Could you check a few things on this model? Use its own coordinates, in mm. A direction names the side the tool comes from. Give positions to 0.01 mm unless a question says otherwise; leave off trailing zeros. Write each loop counter-clockwise with the first axis right and the second up, starting at its lowest first coordinate (ties: lowest second). Pieces come first, ordered by that corner, then holes. Notation, with made-up numbers: (77, -33) -> (88, -33) arc R12 ccw to (88, -14) -> close; hole circle Ø2 at (-37.75, 52). An arc over 180 degrees is marked (long way). One line per question, with ' | ' between items.
from build123d import *

# Parameters (mm, degrees)
F0_W      = 500
F0_H      = 300
F1_DEPTH  = 400
F2_W      = 194.6479137987
F2_H      = 116.2542514503
F2_W_2    = 185.7395432889
F2_H_2    = 104.6733558178
F3_DEPTH  = 200
F4_W      = 200.438356027
F4_H      = 251.2160688639
F4_W_2    = 207.3423415422
F4_H_2    = 244.5347867906
F5_DEPTH  = 200
F6_W      = 311.2314343452
F6_H      = 161.7837399244
F7_DEPTH  = 300
F8_W      = 785.5169922113
F8_H      = 196.2788403034
F9_DEPTH  = 200
F10_DEPTH = 200
F11_W     = 207.3423415422
F11_H     = 178.8012206554
F12_DEPTH = 300
F13_W     = 330.7198137045
F13_H     = 196.2788403034
F14_DEPTH = 700
F15_W     = 178.8012206554
F15_H     = 229.1771650314
F16_DEPTH = 400
F17_W     = 166.0685539246
F17_H     = 392.9448246956
F18_DEPTH = 200
F19_DEPTH = 600
F20_W     = 166.0685539246
F20_H     = 228.0832886696
F21_DEPTH = 230
F22_W     = 230
F22_H     = 228.0832886696
F23_DEPTH = 600
F24_W     = 191.9558256865
F24_H     = 228.0832886696
F25_DEPTH = 600
F26_W     = 330.7198137045
F26_H     = 224.4375318289
F27_DEPTH = 500
F28_W     = 330.7198137045
F28_H     = 150.941491127
F29_DEPTH = 400
F30_W     = 330.7198137045
F30_H     = 173.616194725
F31_DEPTH = 300
F32_W     = 230.9049870819
F32_H     = 232.3303222656
F33_DEPTH = 400
F34_W     = 200
F34_H     = 232.3303222656
F35_DEPTH = 400
F36_W     = 134.3211080879
F36_H     = 232.3303222656
F37_DEPTH = 450
F38_W     = 220.0524806976
F38_H     = 194.8631778359
F39_DEPTH = 1000
F40_W     = 194.8631778359
F40_H     = 226.6708314419
F41_DEPTH = 500
F42_W     = 213.9312028885
F42_H     = 194.8631778359
F43_DEPTH = 300
F44_W     = 213.9312028885
F44_H     = 224.6371984482
F45_DEPTH = 150
F46_W     = 172.431588918
F46_H     = 224.6371984482
F47_DEPTH = 400
F48_R     = 65.9786612065
F49_DEPTH = 100
F50_R     = 50
F51_DEPTH = 100
F52_R     = 50
F53_DEPTH = 200
F54_R     = 50
F55_DEPTH = 200
F56_R     = 50
F57_DEPTH = 200
F58_W     = 1393.2492136955
F58_H     = 511.3118588924
F58_R     = 50
F59_DEPTH = 200


with BuildPart() as f1:
    # F0 (on Front) → F1 (new body)
    with BuildSketch(Plane.XZ):
        with Locations((0, -50)):
            Rectangle(F0_W, F0_H)
    extrude(amount=F1_DEPTH)

    # F2 (on face) → F3 (join)
    with BuildSketch(Plane.XY.offset(100)):
        with Locations((110.0183846429, -98.0239007622)):
            Rectangle(F2_W, F2_H)
        with Locations((-118.4813398868, -227.6407033205)):
            Rectangle(F2_W_2, F2_H_2)
    extrude(amount=F3_DEPTH)

    # F4 (on face) → F5 (join)
    with BuildSketch(Plane.XY.offset(300)):
        with Locations((-111.1319335178, -154.3693467975)):
            Rectangle(F4_W, F4_H)
        with Locations((103.6711707711, -161.2733323127)):
            Rectangle(F4_W_2, F4_H_2)
    extrude(amount=F5_DEPTH)

    # F6 (on face) → F7 (join)
    with BuildSketch(Plane.XZ.offset(400)):
        with Locations((3.1632035971, -80.8918699622)):
            Rectangle(F6_W, F6_H)
    extrude(amount=F7_DEPTH)

    # F8 (on face) → F9 (join)
    with BuildSketch(Plane(origin=(0, -28.7613123655, 0), x_dir=(-1, 0, 0), z_dir=(0, 1, 0))):
        with Locations((-181.4073845744, 401.8605798483)):
            Rectangle(F8_W, F8_H)
    extrude(amount=F9_DEPTH)

    # F10 (add): a face of the model
    f10_faces = [f1.faces().sort_by_distance(p)[0] for p in [
        (103.6711707711, -283.540725708, 400),
    ]]
    extrude(f10_faces, amount=F10_DEPTH)

    # F11 (on face) → F12 (join)
    with BuildSketch(Plane.XY.offset(500)):
        with Locations((103.6711707711, -394.1401153803)):
            Rectangle(F11_W, F11_H)
    extrude(amount=F12_DEPTH)

    # F13 (on face) → F14 (join)
    with BuildSketch(Plane.XZ.offset(28.7613123655)):
        with Locations((408.8059738278, 401.8605798483)):
            Rectangle(F13_W, F13_H)
    extrude(amount=F14_DEPTH)

    # F15 (on face) → F16 (join)
    with BuildSketch(Plane.YZ.offset(207.3423415422)):
        with Locations((-394.1401153803, 685.4114174843)):
            Rectangle(F15_W, F15_H)
    extrude(amount=F16_DEPTH)

    # F17 (on face) → F18 (join)
    with BuildSketch(Plane(origin=(-250, 0, 0), x_dir=(0, -1, 0), z_dir=(-1, 0, 0))):
        with Locations((368.2630956173, -3.5275876522)):
            Rectangle(F17_W, F17_H)
    extrude(amount=F18_DEPTH)

    # F19 (add): a face of the model
    f19_faces = [f1.faces().sort_by_distance(p)[0] for p in [
        (-350, -368.2630956173, 192.9448246956),
    ]]
    extrude(f19_faces, amount=F19_DEPTH)

    # F20 (on face) → F21 (join)
    with BuildSketch(Plane.YZ.offset(-250)):
        with Locations((-368.2630956173, 678.9031803608)):
            Rectangle(F20_W, F20_H)
    extrude(amount=F21_DEPTH)

    # F22 (on face) → F23 (join)
    with BuildSketch(Plane(origin=(0, -285.228818655, 0), x_dir=(-1, 0, 0), z_dir=(0, 1, 0))):
        with Locations((135, 678.9031803608)):
            Rectangle(F22_W, F22_H)
    extrude(amount=F23_DEPTH)

    # F24 (on face) → F25 (join)
    with BuildSketch(Plane.YZ.offset(-20)):
        with Locations((218.7932685018, 678.9031803608)):
            Rectangle(F24_W, F24_H)
    extrude(amount=F25_DEPTH)

    # F26 (on face) → F27 (join)
    with BuildSketch(Plane.XY.offset(500)):
        with Locations((408.8059738278, -616.5425464511)):
            Rectangle(F26_W, F26_H)
    extrude(amount=F27_DEPTH)

    # F28 (on face) → F29 (join)
    with BuildSketch(Plane(origin=(0, -504.3237805367, 0), x_dir=(-1, 0, 0), z_dir=(0, 1, 0))):
        with Locations((-408.8059738278, 924.5292544365)):
            Rectangle(F28_W, F28_H)
    extrude(amount=F29_DEPTH)

    # F30 (on face) → F31 (join)
    with BuildSketch(Plane(origin=(0, 0, 849.058508873), x_dir=(1, 0, 0), z_dir=(0, 0, -1))):
        with Locations((408.8059738278, 191.1318778992)):
            Rectangle(F30_W, F30_H)
    extrude(amount=F31_DEPTH)

    # F32 (on face) → F33 (join)
    with BuildSketch(Plane(origin=(0, 0, 0), x_dir=(-1, 0, 0), z_dir=(0, 1, 0))):
        with Locations((-95.0625883415, -42.5678789616)):
            Rectangle(F32_W, F32_H)
    extrude(amount=F33_DEPTH)

    # F34 (on face) → F35 (join)
    with BuildSketch(Plane(origin=(-20.3899051994, 0, 0), x_dir=(0, -1, 0), z_dir=(-1, 0, 0))):
        with Locations((-300, -42.5678789616)):
            Rectangle(F34_W, F34_H)
    extrude(amount=F35_DEPTH)

    # F36 (on face) → F37 (join)
    with BuildSketch(Plane.XZ.offset(-200)):
        with Locations((-353.2293511555, -42.5678789616)):
            Rectangle(F36_W, F36_H)
    extrude(amount=F37_DEPTH)

    # F38 (on face) → F39 (join)
    with BuildSketch(Plane.XY.offset(73.5972821712)):
        with Locations((-396.0950374603, -152.568411082)):
            Rectangle(F38_W, F38_H)
    extrude(amount=F39_DEPTH)

    # F40 (on face) → F41 (join)
    with BuildSketch(Plane.YZ.offset(-286.0687971115)):
        with Locations((-152.568411082, 960.2618664503)):
            Rectangle(F40_W, F40_H)
    extrude(amount=F41_DEPTH)

    # F42 (on face) → F43 (join)
    with BuildSketch(Plane(origin=(0, 0, 846.9264507294), x_dir=(1, 0, 0), z_dir=(0, 0, -1))):
        with Locations((106.9656014442, 152.568411082)):
            Rectangle(F42_W, F42_H)
    extrude(amount=F43_DEPTH)

    # F44 (on face) → F45 (join)
    with BuildSketch(Plane(origin=(0, -55.1368221641, 0), x_dir=(-1, 0, 0), z_dir=(0, 1, 0))):
        with Locations((-106.9656014442, 659.2450499535)):
            Rectangle(F44_W, F44_H)
    extrude(amount=F45_DEPTH)

    # F46 (on face) → F47 (join)
    with BuildSketch(Plane.YZ.offset(213.9312028885)):
        with Locations((8.647383377, 659.2450499535)):
            Rectangle(F46_W, F46_H)
    extrude(amount=F47_DEPTH)

    # F48 (on face) → F49 (join)
    with BuildSketch(Plane.XZ.offset(700)):
        with Locations((0, -72.7314278483)):
            Circle(F48_R)
    extrude(amount=F49_DEPTH)

    # F50 (on face) → F51 (join)
    with BuildSketch(Plane.YZ.offset(607.3423415422)):
        with Locations((-393.540725708, 680)):
            Circle(F50_R)
    extrude(amount=F51_DEPTH)

    # F52 (on face) → F53 (join)
    with BuildSketch(Plane.YZ.offset(574.1658806801)):
        with Locations((-191.1318778992, 680)):
            Circle(F52_R)
    extrude(amount=F53_DEPTH)

    # F54 (on face) → F55 (join)
    with BuildSketch(Plane.YZ.offset(613.9312028885)):
        with Locations((8.647383377, 680)):
            Circle(F54_R)
    extrude(amount=F55_DEPTH)

    # F56 (on face) → F57 (join)
    with BuildSketch(Plane.YZ.offset(580)):
        with Locations((218.7932685018, 678.9031803608)):
            Circle(F56_R)
    extrude(amount=F57_DEPTH)

    # F58 (on face) → F59 (cut)
    with BuildSketch(Plane.YZ.offset(707.3423415422)):
        with Locations((-61.5827143192, 670.519605279)):
            Rectangle(F58_W, F58_H)
        with Locations((-393.540725708, 680)):
            Circle(F58_R, mode=Mode.SUBTRACT)
    extrude(amount=F59_DEPTH, mode=Mode.SUBTRACT)


solid = f1.part
Q1. Imagine slicing it at B-B on y = 143.5. Please give me the cut outline in (x, z), and give its area (3 significant figures).
Answer below:
outline: (-420.39, -158.73) -> (-286.07, -158.73) -> (-286.07, 73.6) -> (-420.39, 73.6) -> close; (-250, 564.86) -> (580, 564.86) -> (580, 792.94) -> (-250, 792.94) -> close; (-211.35, 303.72) -> (574.17, 303.72) -> (574.17, 500) -> (-211.35, 500) -> close; (-20.39, -158.73) -> (210.52, -158.73) -> (210.52, 73.6) -> (-20.39, 73.6) -> close | area: 428,000 mm^2
Q2. On a 3-axis mill with a long thin cutter (end or side, diameter ignored), from which of +Z, -Z, +X, -X, +Y, -Y can I reach the whole of each face in a straight line? I mean faces 1 (the flat face through (-3, -197, 100)), 2 (the flat face through (-250, -386, 262)), 3 (the flat face through (411, -421, 1000)), 4 (the cylindrical face through (659.983, 2.138, 729.575)), 5 (the flat face through (234, -42, 546.926)). Say none if no direction works.
Answer below:
face 1: none | face 2: -Y | face 3: +Z, +X, +Y, -Y | face 4: +X | face 5: +X, +Y
Q3. If we mould it in two halves opening along Y, with no side actions, what happens to faces 6 (the flat face through (102, -39.006, 399)), 7 (the flat face through (-113, -279.977, 297)), 8 (the flat face through (0, -314, 491))? For each: +Y half, -Y half, draft (parallel to the pull), parting line (faces both ways), or undercut.
Answer below:
face 6: undercut | face 7: -Y half | face 8: draft
Q4. Imagine slicing it at A-A on x = -108. Please give me the cut outline in (y, z).
Answer below:
outline: (-700, -161.78) -> (-400, -161.78) -> (-400, -200) -> (0, -200) -> (0, 100) -> (-175.3, 100) -> (-175.3, 300) -> (-28.76, 300) -> (-28.76, 303.72) -> (171.24, 303.72) -> (171.24, 500) -> (-279.98, 500) -> (-279.98, 100) -> (-400, 100) -> (-400, 0) -> (-700, 0) -> close; (-451.3, 564.86) -> (314.77, 564.86) -> (314.77, 792.94) -> (-451.3, 792.94) -> close; (-250, 846.93) -> (-55.14, 846.93) -> (-55.14, 1073.6) -> (-250, 1073.6) -> close; (200, -158.73) -> (400, -158.73) -> (400, 73.6) -> (200, 73.6) -> close
Q5. Will these pins go through, and if not, where does the flat tip stop? pin 1 (6 mm diameter, centred on x = 107.5, y = 250.5, fed in from +Z); pin 2 (2 mm diameter, centred on x = -115.5, z = 77, fed in from -Y); pin 3 (3 mm diameter, centred on x = -302, z = 349, fed in from +Y).
Answer below:
pin 1: stops at z = 792.94 | pin 2: stops at y = -400 | pin 3: stops at y = -55.14
Q6. If I drill on line 1 along Z through (x, y) = (-225, -123.5); line 2 along Y through (x, z) = (523, 604.5); line 3 along X through (y, z) = (-185.5, 702), over which ranges is the centre line in solid material (lowest first)?
Answer below:
line 1: z = -200 to 100, 564.86 to 792.94, 846.93 to 1073.6 | line 2: y = -728.76 to -504.32, -483.54 to -304.74, -277.94 to -104.32, -77.57 to 94.86, 122.82 to 314.77 | line 3: x = -506.12 to -286.07, -250 to -20, 0 to 213.93, 243.45 to 707.34
